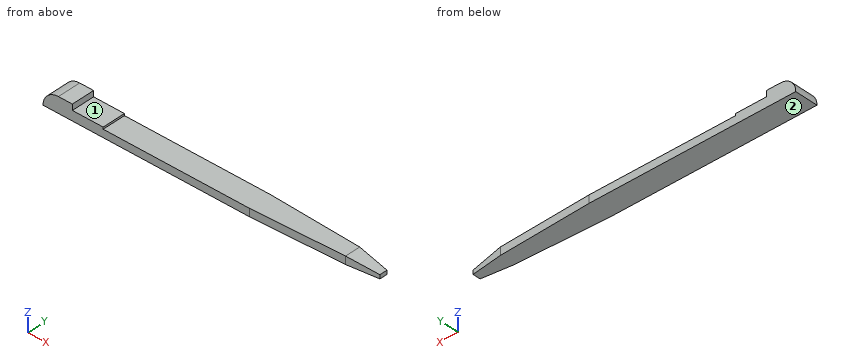
Solid Edge part; units mm, degrees
sketch "Sketch1" plane through (0, 0, 0) normal (0, 0, 1) x (1, 0, 0)
  line L0 (-21.5, -1.5) -> (-21.5, 1.5)
  line L1 (-21.5, 1.5) -> (5.5, 1.5)
  line L2 (5.5, 1.5) -> (17.5, 1)
  line L3 (17.5, 1) -> (21.5, 0.5)
  line L4 (21.5, -0.5) -> (21.5, 0.5)
  line L5 (17.5, -1) -> (21.5, -0.5)
  line L6 (5.5, -1.5) -> (17.5, -1)
  line L7 (5.5, -1.5) -> (-21.5, -1.5)
extrude "Protrusion1" add sketch "Sketch1" against normal blind 1
sketch "Sketch2" plane through (0, 0, 0) normal (0, 0, 1) x (1, 0, 0)
  line L0 (-21.5, 1.5) -> (-17.5, 1.5)
  line L1 (-17.5, -1.5) -> (-17.5, 1.5)
  line L2 (-17.5, -1.5) -> (-21.5, -1.5)
  line L3 (-21.5, -1.5) -> (-21.5, 1.5)
extrude "ExtrudedProtrusion_2" add sketch "Sketch2" along normal blind 1
sketch "Sketch3" plane through (0, 0, 0) normal (0, 0, 1) x (1, 0, 0)
  line L0 (-17.5, -1.5) -> (-17.5, 1.5)
  line L1 (-17.5, 1.5) -> (-13.5, 1.5)
  line L2 (-13.5, 1.5) -> (-13.5, -1.5)
  line L3 (-13.5, -1.5) -> (-17.5, -1.5)
extrude "ExtrudedProtrusion_3" add sketch "Sketch3" along normal blind 0.25
chamfer "Chamfer_1" distance 4 distance2 0.5 1 edges at (21.5, 0, 0) measured on face at (16.0167, -0.97, 0)
sketch "Sketch4" plane through (-8, -1.5, 0) normal (0, -1, 0) x (1, 0, 0)
  line L0 (-13.31, 1) -> (-13.31, -1)
  line L1 (-13.31, -1) -> (-13.5, -1)
  line L2 (-13.5, -1) -> (-13.5, 1)
  line L3 (-13.5, 1) -> (-13.31, 1)
extrude "ExtrudedCutout_1" cut sketch "Sketch4" against normal blind 3
fillet "Round_5" radius 2 1 edges at (-21.31, 0, 1)
Part model, mm, in its own coordinate system. Face numbers are marked on the shaded views. Round coordinates to 2 decimals unless told otherwise and drop trailing zeros. Write each loop counter-clockwise with the first axis right and the second up, starting at its lowest first coordinate (ties: lowest second). Pieces come first, ordered by that corner, then holes. Notation, with made-up numbers: (36, 59.25) -> (88, 59.25) arc R28 ccw to (88, 91.25) -> close; hole circle Ø3 at (-30, -39). An arc over 180 degrees is marked (long way). Return JSON: item names as keys, results as strings. Group by question number.
Q1. Probe L1, parallel to Z at x = 17.5, y = 0.9; L2, parallel to X at y = 0, z = -0.85; L3, parallel to Z at x = -14.5, y = 1.3. List the from-to ranges inside material, lowest first. Write a range as [from, to].
Q2. Saw through at B-B on x = -5.5. Write the cut outline in (y, z).
Q3. Mould opens along Z. For the marked faces 1 and 2 say: pulls with the +Z half, pulls with the -Z half, needs draft (parallel to the pull), parting line crosses it, or undercut.
Q4. Saw through at C-C on x = 18.5. Write the cut outline in (y, z) (3 decimals).
Answer:
{
 "1": {"L1": "[-1, 0]", "L2": "[-21.3, 21.5]", "L3": "[-1, 0.25]"},
 "2": {"outline": "(-1.5, -1) -> (1.5, -1) -> (1.5, 0) -> (-1.5, 0) -> close"},
 "3": {"face 1": "pulls with the +Z half", "face 2": "pulls with the -Z half"},
 "4": {"outline": "(-0.875, -1) -> (0.875, -1) -> (0.875, -0.125) -> (-0.875, -0.125) -> close"}
}
